```python
from build123d import *

# Parameters (mm, degrees)
SKETCH1_W           = 218
SKETCH1_H           = 20
BOSS_EXTRUDE1_DEPTH = 30
SKETCH2_R           = 3.25
CUT_EXTRUDE1_DEPTH  = 30
SKETCH3_R           = 7.475
CUT_EXTRUDE2_DEPTH  = 221.281637909
SKETCH4_R           = 5.7225
CUT_EXTRUDE3_DEPTH  = 15


with BuildPart() as part:
    # Sketch1 → Boss-Extrude1 (new body)
    with BuildSketch(Plane(origin=(0, 0, 0), x_dir=(1, 0, 0), z_dir=(0, 1, 0))):
        Rectangle(SKETCH1_W, SKETCH1_H)
    extrude(amount=BOSS_EXTRUDE1_DEPTH)

    # Sketch2 → Cut-Extrude1 (cut)
    with BuildSketch(Plane.XY.offset(10)):
        with Locations((-72, 24)):
            Circle(SKETCH2_R)
        with Locations((72, 24)):
            Circle(SKETCH2_R)
    extrude(amount=-CUT_EXTRUDE1_DEPTH, mode=Mode.SUBTRACT)

    # Sketch3 → Cut-Extrude2 (cut, through all)
    with BuildSketch(Plane.ZY.offset(109)):
        with Locations((0, 11)):
            Circle(SKETCH3_R)
    extrude(amount=-CUT_EXTRUDE2_DEPTH, mode=Mode.SUBTRACT)

    # Sketch4 → Cut-Extrude3 (cut)
    with BuildSketch(Plane(origin=(0, 30, 0), x_dir=(1, 0, 0), z_dir=(0, 1, 0))):
        with Locations(Location((-90, 0, 0), (0, 0, 270))):
            Circle(SKETCH4_R)
        with Locations(Location((-54, 0, 0), (0, 0, 270))):
            Circle(SKETCH4_R)
        with Locations(Location((-18, 0, 0), (0, 0, 270))):
            Circle(SKETCH4_R)
        with Locations(Location((90, 0, 0), (0, 0, 270))):
            Circle(SKETCH4_R)
        with Locations(Location((18, 0, 0), (0, 0, 270))):
            Circle(SKETCH4_R)
        with Locations(Location((54, 0, 0), (0, 0, 270))):
            Circle(SKETCH4_R)
    extrude(amount=-CUT_EXTRUDE3_DEPTH, mode=Mode.SUBTRACT)


solid = part.part
```
Geometry check sheet. Reference: the model listing, model coordinates, mm. A direction names the side the tool comes from. Round coordinates to 2 decimals unless told otherwise and drop trailing zeros. Loops run counter-clockwise (first coordinate to the right, second up) from the corner with the lowest first, then second, coordinate; pieces in that order, holes last. Notation, with made-up numbers: (70, 0) - (97, 0) arc R24 ccw to (97, 18) - close; hole circle Ø4 at (3.25, 28.25). An arc over 180 degrees is marked (long way). Write item = value, one per line. Start each with the question number.
1. Section check D-D on y = 11. Enter the section's corners in (x, z) (3 decimals).
2. Depth check by flat-ended pin: pin 1 (6 mm diameter, centred on x = -47.5, z = -3, fed in from -Y); pin 2 (1 mm diameter, centred on x = 20.5, z = 1.5, fed in from +Y). Enter the tip coordinate at first touch or a pass-through.
3. Thickness scan on line 1 (X direction, y = 21.5, z = 6.5); line 2 (Y direction, x = -74, z = 3); line 3 (Z direction, x = -90, y = 19). Record the ranges inside material, lowest first.
4. Section check C-C on x = 72. Enter the section's corners in (y, z) (3 decimals).
5. Section check A-A on y = 24. Give the number of separate pieces and of enclosed holes in the cut face, then the cut area to 3 significant figures.
6. Set-up check for faces 1 (the face through (-2, 15, -10)), 2 (the face through (91.719, 23.004, 5.458)): record each of +Z, -Z, +X, -X, +Y, -Y from which the full face is reachable in a straight line by a thin tool's end or side.
7. Mould release check, pull along Y, two halves, no side actions. Record for faces 3 (the face through (-2, 15, 10)), 4 (the face through (-2, 0, 0)), 5 (the face through (-1.5, 3.7, -1.6)): released by +Y, released by -Y, zero draft, split by the parting line, or undercut.
Working result:
q1.outline = (-109, -10) - (109, -10) - (109, -7.475) - (-109, -7.475) - close; (-109, 7.475) - (109, 7.475) - (109, 10) - (-109, 10) - close
q2.pin_1 = 0
q2.pin_2 = 3.8
q3.line_1 = -109 to -74.08, -69.92 to 69.92, 74.08 to 109
q3.line_2 = 0 to 4.15, 17.85 to 21.44, 26.56 to 30
q3.line_3 = -10 to -5.72, 5.72 to 10
q4.outline = (0, -10) - (20.75, -10) - (20.75, 10) - (0, 10) - close; (27.25, -10) - (30, -10) - (30, 10) - (27.25, 10) - close; hole circle Ø14.95 at (11, 0)
q5.separate_pieces = 3
q5.enclosed_holes = 6
q5.area = 3,480 mm^2
q6.face_1 = -Z, +X, -X, +Y, -Y
q6.face_2 = +Y
q7.face_3 = zero draft
q7.face_4 = released by -Y
q7.face_5 = undercut
